from build123d import *

# Parameters (mm, degrees)
F1_DEPTH = 0.3
F2_W     = 50
F2_H     = 80
F3_DEPTH = 1


with BuildPart() as f1:
    # F0 (on Top) → F1 (new body)
    with BuildSketch(Plane.XY):
        Polygon((0.712675, 15.270151), (0.690062, 20.777893), (0, 20.777893), (-6.158038, 18.574403), (-15.406642, 12.183537), (-14.377871, 6.422419), (-15.201324, -3.648944), (-10.119598, -7.209389), (-8.745982, -15.490465), (-6.2484, -16.724988), (-4.502518, -19.434085), (-3.799315, -19.222107), (-4.405524, -11.486877), (-3.435589, -3.363675), (-9.958401, -0.647857), (-10.324874, 3.315877), (-10.173654, 4.244799), (-1.402901, -0.205386), (-1.035653, -0.875074), (-2.202206, -5.822124), (-0.236348, -7.658365), (0.390134, -7.658365), (2.312787, -5.800521), (1.491879, -0.647857), (6.706654, 2.165446), (7.070379, 4.129564), (5.785215, 3.717342), (7.361359, 8.639761), (7.361359, 5.366231), (8.622275, 4.954008), (8.355541, 3.086884), (10.998614, 4.020446), (10.228239, -1.372148), (8.016065, -1.90828), (7.144242, -4.575033), (6.585411, -2.659979), (3.578614, -3.290436), (4.227621, -10.86133), (4.771292, -10.814724), (5.246052, -9.648911), (5.925006, -8.994205), (6.203862, -7.005839), (7.057673, -8.588474), (7.057673, -11.031068), (7.64664, -11.031068), (8.737817, -8.678976), (8.422588, -6.060153), (9.113666, -6.787604), (9.441019, -7.866656), (10.25334, -7.721166), (10.25334, -6.193519), (10.54432, -5.332702), (10.54432, -3.712002), (12.530581, -1.477186), (12.184544, -2.933421), (12.573835, -3.290436), (15.10281, -1.418724), (15.742388, 4.331473), (14.796702, 3.967747), (14.418927, 4.667996), (14.069251, 4.667996), (13.329675, 3.725264), (13.4809, 6.812778), (14.833075, 5.871244), (16.21523, 6.841179), (15.165069, 9.887992), (13.579787, 12.826489), (13.134402, 12.707163), (13.134402, 9.996007), (11.924642, 10.957333), (11.438578, 10.870922), (11.254954, 9.758375), (11.438578, 8.170567), (9.742755, 9.315517), (10.334263, 10.191618), (9.710351, 11.832248), (9.289096, 11.832248), (8.695018, 10.870922), (8.273762, 10.870922), (7.013025, 13.207839), (6.585411, 13.207839), (5.753823, 11.723072), (5.341601, 12.983987), (4.880882, 12.971863), (3.910947, 11.516961), (2.965261, 10.522777), (3.668464, 8.18281), (3.341111, 6.800653), (3.183496, 5.588235), (3.578614, 4.739542), (3.627767, 3.922476), (1.953327, 5.153279), (1.953327, 6.18205), (1.49038, 6.885044), (0.684509, 6.799313), (0.684509, 13.653399), (0.222199, 13.653399), (-1.667038, 11.85499), (-0.577093, 14.071212), align=None)
    extrude(amount=F1_DEPTH)

    # F2 (on face) → F3 (join)
    with BuildSketch(Plane(origin=(0, 0, 0), x_dir=(1, 0, 0), z_dir=(0, 0, -1))):
        Rectangle(F2_W, F2_H)
        Polygon((0.712675, -15.270151), (0.690062, -20.777893), (0, -20.777893), (-6.158038, -18.574403), (-15.406642, -12.183537), (-14.377871, -6.422419), (-15.201324, 3.648944), (-10.119598, 7.209389), (-8.745982, 15.490465), (-6.2484, 16.724988), (-4.502518, 19.434085), (-3.799315, 19.222107), (-4.405524, 11.486877), (-3.435589, 3.363675), (-9.958401, 0.647857), (-10.324874, -3.315877), (-10.173654, -4.244799), (-1.402901, 0.205386), (-1.035653, 0.875074), (-2.202206, 5.822124), (-0.236348, 7.658365), (0.390134, 7.658365), (2.312787, 5.800521), (1.491879, 0.647857), (6.706654, -2.165446), (7.070379, -4.129564), (5.785215, -3.717342), (7.361359, -8.639761), (7.361359, -5.366231), (8.622275, -4.954008), (8.355541, -3.086884), (10.998614, -4.020446), (10.228239, 1.372148), (8.016065, 1.90828), (7.144242, 4.575033), (6.585411, 2.659979), (3.578614, 3.290436), (4.227621, 10.86133), (4.771292, 10.814724), (5.246052, 9.648911), (5.925006, 8.994205), (6.203862, 7.005839), (7.057673, 8.588474), (7.057673, 11.031068), (7.64664, 11.031068), (8.737817, 8.678976), (8.422588, 6.060153), (9.113666, 6.787604), (9.441019, 7.866656), (10.25334, 7.721166), (10.25334, 6.193519), (10.54432, 5.332702), (10.54432, 3.712002), (12.530581, 1.477186), (12.184544, 2.933421), (12.573835, 3.290436), (15.10281, 1.418724), (15.742388, -4.331473), (14.796702, -3.967747), (14.418927, -4.667996), (14.069251, -4.667996), (13.329675, -3.725264), (13.4809, -6.812778), (14.833075, -5.871244), (16.21523, -6.841179), (15.165069, -9.887992), (13.579787, -12.826489), (13.134402, -12.707163), (13.134402, -9.996007), (11.924642, -10.957333), (11.438578, -10.870922), (11.254954, -9.758375), (11.438578, -8.170567), (9.742755, -9.315517), (10.334263, -10.191618), (9.710351, -11.832248), (9.289096, -11.832248), (8.695018, -10.870922), (8.273762, -10.870922), (7.013025, -13.207839), (6.585411, -13.207839), (5.753823, -11.723072), (5.341601, -12.983987), (4.880882, -12.971863), (3.910947, -11.516961), (2.965261, -10.522777), (3.668464, -8.18281), (3.341111, -6.800653), (3.183496, -5.588235), (3.578614, -4.739542), (3.627767, -3.922476), (1.953327, -5.153279), (1.953327, -6.18205), (1.49038, -6.885044), (0.684509, -6.799313), (0.684509, -13.653399), (0.222199, -13.653399), (-1.667038, -11.85499), (-0.577093, -14.071212), align=None, mode=Mode.SUBTRACT)
    extrude(amount=-F3_DEPTH)


solid = f1.part
Can you work these out from the model? Positions are in its coordinate system, mm. A direction names the side the tool comes from. Give positions to 0.01 mm unless a question says otherwise; leave off trailing zeros. Loops run counter-clockwise (first coordinate to the right, second up) from the corner with the lowest first, then second, coordinate; pieces in that order, holes last. Notation, with made-up numbers: M 22.25,4 L 51.25,4 A11 ccw 51.25,18 Z; hole C -3.5,33 d1. An arc over 180 degrees is marked long. One line per item, written item: value.
1) Imagine slicing it at A-A on y = 20. Write out the boundary of the cut face in (x, z).
Geometry check:
outline: M -25,0 L 25,0 L 25,1 L 0.69,1 L 0.69,0.3 L -2.17,0.3 L -2.17,1 L -25,1 Z
2) Imagine slicing it at B-B on y = -13.5. Write out the boundary of the cut face in (x, z).
Geometry check:
outline: M -25,0 L 25,0 L 25,1 L -4.25,1 L -4.25,0.3 L -9.08,0.3 L -9.08,1 L -25,1 Z
3) On a 3-axis mill with a long thin cutter (end or side, diameter ignored), from which of +Z, -Z, +X, -X, +Y, -Y can I reach the whole of each face in a straight line? I mean faces 3 (the face through (-3.04, 19.69, 0.65)), 4 (the face through (5, -1, 1)). Say none if no direction works.
Geometry check:
face 3: +Z
face 4: +Z, +X, -X, +Y, -Y
4) Thinking about a two-plate mould opening in X: for faces 1 (the face through (13.82, -2.37, 0.65)), 2 (the face through (0, -1, 0)), which applies, +X half, -X half, draft (parallel to the pull), parting line (faces both ways), or undercut?
Geometry check:
face 1: undercut
face 2: draft
5) Please list where these lines run through material, in increasing order: line 1 (X direction, y = 2, z = 0.9); line 2 (X direction, y = -9.5, z = 0.6); line 3 (Y direction, x = -4.5, z = 0.35).
Geometry check:
line 1: x = -25 to -14.74, -10.2 to -5.75, 6.4 to 10.71, 15.48 to 25
line 2: x = -25 to -9.74, -4.17 to 4.11, 5.4 to 7.06, 8.36 to 25
line 3: y = -40 to -19.43, -2.92 to 1.37, 19.17 to 40
